The model under review builds one solid part; all positions refer to its coordinate system, in mm. A direction names the side the tool comes from. Give positions to 0.01 mm unless a question says otherwise; leave off trailing zeros. Loops run counter-clockwise (first coordinate to the right, second up) from the corner with the lowest first, then second, coordinate; pieces in that order, holes last. Notation, with made-up numbers: M 49.5,43 L 103.5,43 A23 ccw 103.5,55 Z; hole C -14,11 d8. An arc over 180 degrees is marked long. Put each result on its own line as item: value. Start each with the question number.
Autodesk Inventor part; units mm, degrees
ref_plane "YZ Plane" through (0, 0, 0) normal (1, 0, 0) x (0, 1, 0)
ref_plane "XZ Plane" through (0, 0, 0) normal (0, 1, 0) x (-1, 0, 0)
ref_plane "XY Plane" through (0, 0, 0) normal (0, 0, 1) x (1, 0, 0)
sketch "草图1" plane through (0, 0, 0) normal (0, 0, 1) x (1, 0, 0)
  circle A0 centre (0, 0) radius 5
  dimension "d0" = 10
extrude "拉伸1" add sketch "草图1" along normal blind 5
sketch "草图2" plane through (0, 0, 5) normal (0, 0, 1) x (1, 0, 0)
  circle A0 centre (0, 0) radius 5
  circle A1 centre (0, 0) radius 5
  line L0 (1.7321, -3) -> (-1.7321, -3)
  line L1 (-1.7321, -3) -> (-3.4641, 0)
  line L2 (-3.4641, 0) -> (-1.7321, 3)
  line L3 (-1.7321, 3) -> (1.7321, 3)
  line L4 (1.7321, 3) -> (3.4641, 0)
  line L5 (3.4641, 0) -> (1.7321, -3)
  line L6 (0, 0) -> (0, 1.0367)
  point P0 (0, 3)
  dimension "d3" = 1.0367
  dimension "d4" = 6
extrude "拉伸2" cut sketch "草图2" against normal blind 4
fillet "圆角1" radius 0.25 13 edges at (-5, 0, 1) (1.7321, 3, 3) (-2.5981, 1.5, 5) (0, 3, 5) (-1.7321, 3, 3) (-3.4641, 0, 3) (-2.5981, -1.5, 5) (-1.7321, -3, 3) (0, -3, 5) (2.5981, -1.5, 5) (1.7321, -3, 3) (3.4641, 0, 3) (2.5981, 1.5, 5)
sketch "草图3" plane through (0, 0, 0) normal (0, 0, -1) x (-1, 0, 0)
  circle A0 centre (0, 0) radius 2.5
  dimension "d8" = 5
extrude "拉伸3" add sketch "草图3" along normal blind 15
thread "螺纹1"
chamfer "倒角1" distance 0.225 angle 45 1 edges at (2.5, 0, -15)
properties part number "载板下弹片固定螺丝"
(1) We need section A-A, the plane z = 1.25. Write out the cut boundary in (x, y) (3 decimals).
(2) We need section C-C, the plane z = -12.5. Write out the cut boundary in (x, y).
(3) To check wall thickness, follow L1, parallel to Z at x = 3.5, y = 0; L2, parallel to Y at x = 0, z = -13.25; L3, parallel to Z at x = 2.75, y = -0.5. State the ranges of each line that lie inside material, in increasing order. Write a range as [from, to].
(4) For faces 1 (the flat face through (-2.6, 1.5, 2.9)), 2 (the cylindrical face through (0.54, 2.44, -7.28)), 3 (the flat face through (0, 3, 3)), 4 (the flat face through (2.6, -1.5, 2.9)), 5 (the flat face through (3.1, -1, 1)), list the 3-axis set-ups (+Z, -Z, +X, -X, +Y, -Y) from which the entire face can be reached by the end or side of a thin tool; tool diameter is ignored.
(5) Insertion check: pin 1 (2.5 mm diameter, centred on x = 0, z = 3.5, fed in from +Y); pin 2 (1.5 mm diameter, centred on x = 3, z = 1, fed in from -Y); pin 3 (5 mm diameter, centred on x = 1.5, z = -12.5, fed in from +Y); pin 4 (1 mm diameter, centred on x = 3.5, y = -0.5, fed in from +Z). Each pin has a flat end and moves straight along its axis. Give the tip position at first contact, or say it passes through.
(6) We need section B-B, the plane x = 0. Write out the cut boundary in (y, z) (3 decimals).
Check sheet entries:
1. outline: M -3.392,-0.125 L -1.804,-2.875 A0.25 ccw -1.588,-3 L 1.588,-3 A0.25 ccw 1.804,-2.875 L 3.392,-0.125 A0.25 ccw 3.392,0.125 L 1.804,2.875 A0.25 ccw 1.588,3 L -1.588,3 A0.25 ccw -1.804,2.875 L -3.392,0.125 A0.25 ccw Z
2. outline: C 0,0 d5
3. L1: z = [0, 1]
3. L2: y = [-2.5, 2.5]
3. L3: z = [0, 5]
4. face 1: +Z, -X, +Y
4. face 2: -Z
4. face 3: +Z, +X, -X, +Y
4. face 4: +Z, +X, -Y
4. face 5: +Z
5. pin 1: stops at y = 3
5. pin 2: stops at y = -4.45
5. pin 3: stops at y = 2.5
5. pin 4: stops at z = 5
6. outline: M -5,0 L -2.5,0 L -2.5,-14.775 L -2.275,-15 L 2.275,-15 L 2.5,-14.775 L 2.5,0 L 5,0 L 5,0.75 A0.25 ccw 4.75,1 L 3,1 L 3,4.75 A0.25 ccw 2.75,5 L -2.75,5 A0.25 ccw -3,4.75 L -3,1 L -4.75,1 A0.25 ccw -5,0.75 Z
